Source: CAD feature listing. Evaluate the final solid. Frame: model axes, mm. Face numbers are marked on the shaded views. A direction names the side the tool comes from. Give positions to 0.01 mm unless a question says otherwise; leave off trailing zeros. Order: outer loops, then holes, each group sorted by start corner. A loop starts at its lowest first (then second) coordinate and runs counter-clockwise, first axis right, second up.
1) Section A-A, the plane x = 10.1. Return loops of the section in (y, z).
2) First-contact query: P1, Ø1.5, axis at y = 37, z = 25, coming from the +X side; P2, Ø1.5, axis at y = 48.5, z = 24, coming from the +X side; P3, Ø1.5, axis at x = -3, z = 24.5, coming from the -Y side. Flat tips, straight axial feed; report the tip coordinate or a pass-through.
3) Material intervals for line 1 (X direction, y = 18.5, z = 23.6); line 2 (X direction, y = 8, z = 24.85); line 3 (Y direction, x = -3.69, z = 23.7), sorted ascending.
4) Draft query along Y for the marked faces 3, 4, 5 and 6. Return one class per face: released by +Y, released by -Y, zero draft, split by the parting line, or undercut.
5) Section B-B, the plane y = 14.5. Return loops of the section in (x, z).
6) Section C-C, the plane z = 23.9. Return loops of the section in (x, y), plus the area to 3 significant figures.
7) Section D-D, the plane y = 5. Return loops of the section in (x, z).
8) Access query for the marked faces 1 and 2. Directions: +Z, -Z, +X, -X, +Y, -Y. A direction counts if a zero-diameter tool reaches every point of the face in a straight line with its end or side. Return the directions, or none.
```python
from build123d import *

# Parameters (mm, degrees)
SKETCH1_R           = 2
BOSS_EXTRUDE1_DEPTH = 3


with BuildPart() as part:
    # Sketch1 → Boss-Extrude1 (new body)
    with BuildSketch(Plane.XY.offset(26)):
        with BuildLine():
            Line((0, 0), (20.2, 0))
            Line((20.2, 0), (20.2, 18.206774978))
            ThreePointArc((20.2, 18.206774978), (21.746211994, 23.548447782), (25.906693669, 27.238248874))
            ThreePointArc((25.906693669, 27.238248874), (28.587297404, 31.480600764), (25.906693669, 35.722952653))
            ThreePointArc((25.906693669, 35.722952653), (21.746211994, 39.412753746), (20.2, 44.754426549))
            Line((20.2, 44.754426549), (20.2, 52.179630025))
            ThreePointArc((20.2, 52.179630025), (10.1, 55.643160629), (0, 52.179630025))
            Line((0, 52.179630025), (0, 45.258439456))
            ThreePointArc((0, 45.258439456), (-1.571872489, 39.876370461), (-5.793333333, 36.186286704))
            ThreePointArc((-5.793333333, 36.186286704), (-8.69, 31.650210328), (-5.793333333, 27.114133952))
            ThreePointArc((-5.793333333, 27.114133952), (-1.571872489, 23.424050195), (0, 18.0419812))
            Line((0, 18.0419812), (0, 0))
        make_face()
        with Locations((-3.69, 31.650210328)):
            Circle(SKETCH1_R, mode=Mode.SUBTRACT)
        with Locations((23.89, 31.480600764)):
            Circle(SKETCH1_R, mode=Mode.SUBTRACT)
        with BuildLine():
            Line((15.15, 12), (15.15, 47.222342094))
            ThreePointArc((15.15, 47.222342094), (10.1, 52.272342094), (5.05, 47.222342094))
            Line((5.05, 47.222342094), (5.05, 12))
            ThreePointArc((5.05, 12), (10.1, 6.95), (15.15, 12))
        make_face(mode=Mode.SUBTRACT)
    extrude(amount=-BOSS_EXTRUDE1_DEPTH)


solid = part.part
```
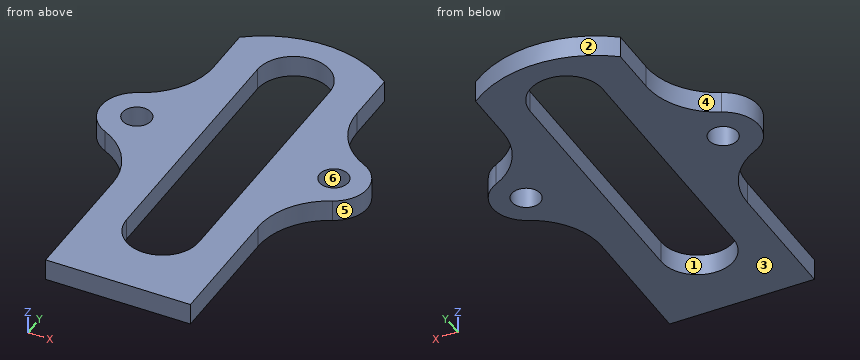
From the geometry:
1. outline: (0, 23) - (6.95, 23) - (6.95, 26) - (0, 26) - close; (52.27, 23) - (55.64, 23) - (55.64, 26) - (52.27, 26) - close
2. P1: stops at x = 24.94
2. P2: stops at x = 20.2
2. P3: stops at y = 24.36
3. line 1: x = -0.01 to 5.05, 15.15 to 20.2
3. line 2: x = 0 to 7.02, 13.18 to 20.2
3. line 3: y = 25.8 to 29.65, 33.65 to 37.5
4. face 3: zero draft
4. face 4: released by +Y
4. face 5: split by the parting line
4. face 6: undercut
5. outline: (0, 23) - (5.05, 23) - (5.05, 26) - (0, 26) - close; (15.15, 23) - (20.2, 23) - (20.2, 26) - (15.15, 26) - close
6. outline: (-5.79, 27.11) arc R10 cw to (0, 18.04) - (0, 0) - (20.2, 0) - (20.2, 18.21) arc R10 cw to (25.91, 27.24) arc R4.7 ccw to (25.91, 35.72) arc R10 cw to (20.2, 44.75) - (20.2, 52.18) arc R16.46 ccw to (0, 52.18) - (0, 45.26) arc R10 cw to (-5.79, 36.19) arc R5 ccw to start; hole circle Ø4 at (-3.69, 31.65); hole (5.05, 12) arc R5.05 ccw to (15.15, 12) - (15.15, 47.22) arc R5.05 ccw to (5.05, 47.22) - close; hole circle Ø4 at (23.89, 31.48)
6. area: 836 mm2
7. outline: (0, 23) - (20.2, 23) - (20.2, 26) - (0, 26) - close
8. face 1: +Z, -Z
8. face 2: +Z, -Z, +Y
